Read the model definition and answer for the solid it produces. Units are mm, in the model's axes. A direction names the side the tool comes from. Give positions to 0.01 mm unless a question says otherwise; leave off trailing zeros. Loops run counter-clockwise (first coordinate to the right, second up) from the corner with the lowest first, then second, coordinate; pieces in that order, holes last. Notation, with made-up numbers: (23, -23.75) - (41, -23.75) arc R35 ccw to (41, 8.25) - close; hole circle Ø4 at (74, 53). An arc over 180 degrees is marked (long way). Use a Markdown table: item, result. Add a question column.
Item 1: A cutting plane is placed at A-A (x = -15). Determine the outline of the cut face in (y, z) (3 decimals), plus the area to 3 significant figures.
Item 2: Which of the six approach directions +Z, -Z, +X, -X, +Y, -Y give full straight-line access (tool end or side, diameter ignored) to faces 4 (the face through (-25, 49, 2)), 5 (the face through (10, 80, 2)), 6 (the face through (20, 20, 2)), 7 (the face through (-25, 20, 2)), 8 (the face through (10, 0, 2))?
Item 3: A cutting plane is placed at B-B (z = 0.5). Give the number of separate pieces and of enclosed holes in the cut face, plus the area to 3 significant figures.
Item 4: For a pull along Y with two mould halves and no side action, classify faces 1 (the face through (18.38, 6.27, 1.57)), 2 (the face through (12, 41, 3.175)), 3 (the face through (-30.037, 34.797, 1.565)) as +Y half, -Y half, draft (parallel to the pull), parting line (faces both ways), or undercut.
Item 5: A cutting plane is placed at D-D (x = 3). Determine the outline of the cut face in (y, z) (3 decimals), plus the area to 3 significant figures.
Item 6: Each of these flat-tipped pins is pushed along its axis until it touches: P1, Ø1, axis at x = 37.5, z = 2.5, coming from the +Y side; P2, Ø1.6, axis at y = 18, z = 1.5, coming from the +X side; P3, Ø1.1, axis at y = 49, z = 1, coming from the -X side. Where does it stop, or does it pass through?
Item 7: Consider probe 1 along Y at (x, z) = (-15, 1.3) (3 decimals); probe 2 along Y at (x, z) = (17, 2.35) (3 decimals); probe 3 along X at (y, z) = (5.5, 1.15). Determine where each line is inside the solid, lowest interval first. Write a range as [from, to].
Item 8: A cutting plane is placed at C-C (y = 68). Determine the outline of the cut face in (x, z) (3 decimals).
from build123d import *

# Parameters (mm, degrees)
BASE_FLANGE1_DEPTH         = 3.175
M3_5_CLEARANCE_HOLE1_D     = 3.75
F_5_2_5_2_DIAMETER_HOLE1_D = 5.2
F_4_2_4_2_DIAMETER_HOLE1_D = 4.2
F_22_0_22_DIAMETER_HOLE1_D = 22


# Sheet-metal steps are written as plain solids
with BuildPart() as part:
    # Sketch11 → Base-Flange1 (new body)
    with BuildSketch(Plane(origin=(0, 0, 0), x_dir=(-1, 0, 0), z_dir=(0, 0, -1))):
        with BuildLine():
            Line((20, 55.487), (5, 55.487))
            ThreePointArc((5, 55.487), (1.464466094, 56.951466094), (0, 60.487))
            Line((0, 60.487), (0, 75))
            ThreePointArc((0, 75), (-1.464466094, 78.535533906), (-5, 80))
            Line((-5, 80), (-15, 80))
            ThreePointArc((-15, 80), (-18.535533906, 78.535533906), (-20, 75))
            Line((-20, 75), (-20, 55))
            Line((-20, 55), (-48, 55))
            ThreePointArc((-48, 55), (-51.535533906, 53.535533906), (-53, 50))
            Line((-53, 50), (-53, 40))
            ThreePointArc((-53, 40), (-51.535533906, 36.464466094), (-48, 35))
            Line((-48, 35), (-20, 35))
            Line((-20, 35), (-20, 5))
            ThreePointArc((-20, 5), (-18.535533906, 1.464466094), (-15, 0))
            Line((-15, 0), (-5, 0))
            ThreePointArc((-5, 0), (-1.464466094, 1.464466094), (0, 5))
            Line((0, 5), (0, 9.287))
            ThreePointArc((0, 9.287), (1.464466094, 12.822533906), (5, 14.287))
            Line((5, 14.287), (20, 14.287))
            ThreePointArc((20, 14.287), (23.535533906, 15.751466094), (25, 19.287))
            Line((25, 19.287), (25, 21.728499788))
            ThreePointArc((25, 21.728499788), (30.037804903, 35), (25, 48.271500212))
            Line((25, 48.271500212), (25, 50.487))
            ThreePointArc((25, 50.487), (23.535533906, 54.022533906), (20, 55.487))
        make_face()
    extrude(amount=-BASE_FLANGE1_DEPTH)

    # M3.5 Clearance Hole1 (through all)
    with Locations(Plane.XY.offset(3.175)):
        with Locations((17, 5), (3, 75), (3, 5), (17, 75)):
            Hole(M3_5_CLEARANCE_HOLE1_D / 2)

    # Ø5.2 (5.2) Diameter Hole1 (through all)
    with Locations(Plane.XY.offset(3.175)):
        with Locations((27.5, 45), (47.5, 45)):
            Hole(F_5_2_5_2_DIAMETER_HOLE1_D / 2)

    # Ø4.2 (4.2) Diameter Hole1 (through all)
    with Locations(Plane.XY.offset(3.175)):
        with Locations((-15, 19.287), (-15, 50.275)):
            Hole(F_4_2_4_2_DIAMETER_HOLE1_D / 2)

    # Ø22.0 (22) Diameter Hole1 (through all)
    with Locations(Plane.XY.offset(3.175)):
        with Locations((-15, 35)):
            Hole(F_22_0_22_DIAMETER_HOLE1_D / 2)


solid = part.part
Geometry says:
| question | item | result |
|---|---|---|
| 1 | outline | (14.287, 0) - (17.187, 0) - (17.187, 3.175) - (14.287, 3.175) - close; (21.387, 0) - (24, 0) - (24, 3.175) - (21.387, 3.175) - close; (46, 0) - (48.175, 0) - (48.175, 3.175) - (46, 3.175) - close; (52.375, 0) - (55.487, 0) - (55.487, 3.175) - (52.375, 3.175) - close |
| 1 | area | 34.3 mm² |
| 2 | face 4 | +Z, -Z, -X, +Y |
| 2 | face 5 | +Z, -Z, +X, -X, +Y |
| 2 | face 6 | +Z, -Z, +X, -Y |
| 2 | face 7 | +Z, -Z, -X, -Y |
| 2 | face 8 | +Z, -Z, +X, -X, -Y |
| 3 | separate pieces | 1 |
| 3 | enclosed holes | 9 |
| 3 | area | 2,850 mm² |
| 4 | face 1 | undercut |
| 4 | face 2 | draft |
| 4 | face 3 | parting line |
| 5 | outline | (0.417, 0) - (3.125, 0) - (3.125, 3.175) - (0.417, 3.175) - close; (6.875, 0) - (73.125, 0) - (73.125, 3.175) - (6.875, 3.175) - close; (76.875, 0) - (79.583, 0) - (79.583, 3.175) - (76.875, 3.175) - close |
| 5 | area | 228 mm² |
| 6 | P1 | y = 55 |
| 6 | P2 | x = 20 |
| 6 | P3 | x = -25 |
| 7 | probe 1 | [14.287, 17.187], [21.387, 24], [46, 48.175], [52.375, 55.487] |
| 7 | probe 2 | [0.417, 3.125], [6.875, 73.125], [76.875, 79.583] |
| 7 | probe 3 | [0, 1.19], [4.81, 15.19], [18.81, 20] |
| 8 | outline | (0, 0) - (20, 0) - (20, 3.175) - (0, 3.175) - close |
